Model file for the job. Use its own axes, mm. A direction names the side the tool comes from. Round coordinates to 2 decimals unless told otherwise and drop trailing zeros. Order: outer loops, then holes, each group sorted by start corner. A loop starts at its lowest first (then second) coordinate and runs counter-clockwise, first axis right, second up. Notation, with made-up numbers: (-37.5, 4.25) -> (-21.5, 4.25) arc R12 cw to (-21.5, 13.25) -> close; hole circle Ø9 at (63.5, -25). An arc over 180 degrees is marked (long way). Answer as CSV lines item,"result".
```python
from build123d import *

# Parameters (mm, degrees)
BOSS_EXTRUDE1_DEPTH = 5
SKETCH2_R           = 2.5
SKETCH2_R_2         = 1.5
SKETCH2_R_3         = 15
CUT_EXTRUDE1_DEPTH  = 5
SKETCH3_R           = 2.5
CUT_EXTRUDE2_DEPTH  = 5
SKETCH4_R           = 23.5
SKETCH4_R_2         = 21.000952359
BOSS_EXTRUDE2_DEPTH = 7
SKETCH5_R           = 30.000666659
SKETCH5_R_2         = 23.5
BOSS_EXTRUDE3_DEPTH = 18


with BuildPart() as part:
    # Sketch1 → Boss-Extrude1 (new body)
    with BuildSketch(Plane(origin=(0, 0, 0), x_dir=(1, 0, 0), z_dir=(0, 1, 0))):
        with BuildLine():
            Line((0, 37), (143.3, 37))
            ThreePointArc((143.3, 37), (180.3, 0), (143.3, -37))
            Line((143.3, -37), (0, -37))
            ThreePointArc((0, -37), (-37, 0), (0, 37))
        make_face()
    extrude(amount=BOSS_EXTRUDE1_DEPTH)

    # Sketch2 → Cut-Extrude1 (cut)
    with BuildSketch(Plane(origin=(0, 5, 0), x_dir=(1, 0, 0), z_dir=(0, 1, 0))):
        with Locations(Location((0, 0, 0), (0, 0, 270))):
            Circle(SKETCH2_R)
        with Locations(Location((-15.5, 15.5, 0), (0, 0, 270))):
            Circle(SKETCH2_R_2)
        with Locations(Location((15.5, 15.5, 0), (0, 0, 270))):
            Circle(SKETCH2_R_2)
        with Locations(Location((15.5, -15.5, 0), (0, 0, 270))):
            Circle(SKETCH2_R_2)
        with Locations(Location((-15.5, -15.5, 0), (0, 0, 270))):
            Circle(SKETCH2_R_2)
        with Locations(Location((143.3, 0, 0), (0, 0, 270))):
            Circle(SKETCH2_R_3)
    extrude(amount=-CUT_EXTRUDE1_DEPTH, mode=Mode.SUBTRACT)

    # Sketch3 → Cut-Extrude2 (cut)
    with BuildSketch(Plane(origin=(0, 5, 0), x_dir=(1, 0, 0), z_dir=(0, 1, 0))):
        with Locations(Location((-31.5, 0, 0), (0, 0, 270))):
            Circle(SKETCH3_R)
        with Locations(Location((4.5, -29, 0), (0, 0, 270))):
            Circle(SKETCH3_R)
        with Locations(Location((38.5, -29, 0), (0, 0, 270))):
            Circle(SKETCH3_R)
        with Locations(Location((72.5, -29, 0), (0, 0, 270))):
            Circle(SKETCH3_R)
        with Locations(Location((106.5, -29, 0), (0, 0, 270))):
            Circle(SKETCH3_R)
        with Locations(Location((4.5, 29, 0), (0, 0, 270))):
            Circle(SKETCH3_R)
        with Locations(Location((38.5, 29, 0), (0, 0, 270))):
            Circle(SKETCH3_R)
        with Locations(Location((72.5, 29, 0), (0, 0, 270))):
            Circle(SKETCH3_R)
        with Locations(Location((106.5, 29, 0), (0, 0, 270))):
            Circle(SKETCH3_R)
    extrude(amount=-CUT_EXTRUDE2_DEPTH, mode=Mode.SUBTRACT)

    # Sketch4 → Boss-Extrude2 (add)
    with BuildSketch(Plane(origin=(0, 5, 0), x_dir=(1, 0, 0), z_dir=(0, 1, 0))):
        with Locations(Location((143.3, 0, 0), (0, 0, 270))):
            Circle(SKETCH4_R)
        with Locations(Location((143.3, 0, 0), (0, 0, 270))):
            Circle(SKETCH4_R_2, mode=Mode.SUBTRACT)
    extrude(amount=BOSS_EXTRUDE2_DEPTH)

    # Sketch5 → Boss-Extrude3 (add)
    with BuildSketch(Plane(origin=(0, 5, 0), x_dir=(1, 0, 0), z_dir=(0, 1, 0))):
        with Locations(Location((143.3, 0, 0), (0, 0, 90))):
            Circle(SKETCH5_R)
        with Locations(Location((143.3, 0, 0), (0, 0, 270))):
            Circle(SKETCH5_R_2, mode=Mode.SUBTRACT)
    extrude(amount=BOSS_EXTRUDE3_DEPTH)


solid = part.part
```
Q1. Saw through at B-B (z = 0). Write the cut outline in (x, y).
Checks:
outline,"(-37, 0) -> (-34, 0) -> (-34, 5) -> (-37, 5) -> close; (-29, 0) -> (-2.5, 0) -> (-2.5, 5) -> (-29, 5) -> close; (2.5, 0) -> (128.3, 0) -> (128.3, 5) -> (122.3, 5) -> (122.3, 12) -> (119.8, 12) -> (119.8, 23) -> (113.3, 23) -> (113.3, 5) -> (2.5, 5) -> close; (158.3, 0) -> (180.3, 0) -> (180.3, 5) -> (173.3, 5) -> (173.3, 23) -> (166.8, 23) -> (166.8, 12) -> (164.3, 12) -> (164.3, 5) -> (158.3, 5) -> close"
Q2. Saw through at D-D (z = -11). Write the cut outline in (x, y).
Checks:
outline,"(-35.33, 0) -> (133.1, 0) -> (133.1, 5) -> (125.41, 5) -> (125.41, 12) -> (122.53, 12) -> (122.53, 23) -> (115.39, 23) -> (115.39, 5) -> (-35.33, 5) -> close; (153.5, 0) -> (178.63, 0) -> (178.63, 5) -> (171.21, 5) -> (171.21, 23) -> (164.07, 23) -> (164.07, 12) -> (161.19, 12) -> (161.19, 5) -> (153.5, 5) -> close"
Q3. Saw through at A-A (x = 72.5). Write the cut outline in (y, z), plus the area to 3 significant figures.
Checks:
outline,"(0, -37) -> (5, -37) -> (5, -31.5) -> (0, -31.5) -> close; (0, -26.5) -> (5, -26.5) -> (5, 26.5) -> (0, 26.5) -> close; (0, 31.5) -> (5, 31.5) -> (5, 37) -> (0, 37) -> close"
area,"320 mm²"
Q4. Mould opens along Z. For faces 1 (the cylindrical face through (109, 3, -29)), 2 (the cylindrical face through (180.29, 2.46, -0.81)), 3 (the flat face through (49, 5, -1)), 4 (the cylindrical face through (36.06, 2.54, 28.46)) say: +Z half, -Z half, draft (parallel to the pull), parting line (faces both ways), or undercut.
Checks:
face 1,"undercut"
face 2,"parting line"
face 3,"draft"
face 4,"undercut"
Q5. Flat gauge pins, fed straight in: pin 1 (10 mm diameter, centred on x = -5.5, z = 14.5, fed in from +Y); pin 2 (6.5 mm diameter, centred on x = 38.5, z = 29, fed in from -Y); pin 3 (6 mm diameter, centred on x = 151.5, y = 16, fed in from -Z); pin 4 (1.5 mm diameter, centred on y = 3, z = -13, fed in from +X). Where does each tip first touch, or does it go through?
Checks:
pin 1,"y = 5"
pin 2,"y = 0"
pin 3,"z = -29.55"
pin 4,"x = 178.21"
Q6. Tool access for faces 5 (the cylindrical face through (166.6, 17.42, -3.06)), 6 (the flat face through (71, 2, -37)): list every direction of +Z, -Z, +X, -X, +Y, -Y with a clear straight run to the whole face (end or side of a thin tool).
Checks:
face 5,"+Y"
face 6,"-Z, +X, -X, +Y, -Y"
Q7. Wall check: L1, parallel to X at y = 3.75, z = 0; L2, parallel to X at y = 1.5, z = -29; L3, parallel to X at y = 19.5, z = 0. Give the ranges that are in metal, low to high. Write a range as [from, to].
Checks:
L1,"[-37, -34], [-29, -2.5], [2.5, 128.3], [158.3, 180.3]"
L2,"[-22.98, 2], [7, 36], [41, 70], [75, 104], [109, 166.28]"
L3,"[113.3, 119.8], [166.8, 173.3]"
Q8. Saw through at C-C (y = 2). State how many separate pieces and enclosed holes the cut face has, plus the area to 3 significant figures.
Checks:
separate pieces,"1"
enclosed holes,"15"
area,"14,000 mm²"
